```python
from build123d import *

# Parameters (mm, degrees)
EXTRUDE_1_DEPTH = 8


with BuildPart() as part:
    # 草图1 → 凸台-拉伸1 (new body)
    with BuildSketch(Plane.XY):
        with BuildLine():
            Line((9.884140627, 48.890967478), (9.862592606, 71.797167618))
            Line((9.862592606, 71.797167618), (9.862592606, 74.789638905))
            Line((9.862592606, 74.789638905), (1.859342158, 74.789638905))
            Line((1.859342158, 74.789638905), (1.859342158, 71.789638905))
            Line((1.859342158, 71.789638905), (1.880609299, 49.182021359))
            add(Edge.make_bspline(
                [(1.880609299, 49.182021359), (-2.147543525, 51.320103541), (-9.368620539, 54.40588996), (-18.684466246, 60.920686929), (-26.75654301, 68.367940859), (-36.33720868, 82.740540116), (-36.066485806, 97.042827626), (-36.847635358, 105.899002406)],
                knots=[0, 0, 0, 0, 0.18493282, 0.316628253, 0.458400557, 0.629057108, 1, 1, 1, 1], degree=3))
            Line((-36.847635358, 105.899002406), (47.833660698, 106.415821201))
            add(Edge.make_bspline(
                [(47.833660698, 106.415821201), (48.319473241, 99.869034947), (47.370463287, 91.039903293), (45.267329493, 80.35246618), (41.497074055, 73.927784135), (37.087778724, 67.31022324), (26.486440292, 57.93257211), (16.797369064, 52.799383097), (9.884140627, 48.890967478)],
                knots=[0, 0, 0, 0, 0.262570007, 0.359675169, 0.434109376, 0.560787033, 0.678988213, 1, 1, 1, 1], degree=3))
        make_face()
    extrude(amount=EXTRUDE_1_DEPTH)


solid = part.part
```
Verification items for the finished model (mm, model axes). Give positions to 0.01 mm unless a question says otherwise; leave off trailing zeros. Answer in a Markdown table with one row per item. Add a question column.
Item 1: Mould release check, pull along X, two halves, no side actions. Record for faces 1 (the flat face through (6, 74.79, 4)), 2 (the flat face through (6, 84, 8)): released by +X, released by -X, zero draft, split by the parting line, or undercut.
Item 2: Scan lines: probe 1 along X at (y, z) = (57, 2); probe 2 along X at (y, z) = (59, 3.75); probe 3 along X at (y, z) = (90, 6.5). Record each from-to range of solid material in increasing order. Write a range as from..to.
Item 3: Gauge pin test, flat ends, axial feed: pin 1 (0.9 mm diameter, centred on y = 73, z = 4, fed in from -X) (3 decimals); pin 2 (1.5 mm diameter, centred on y = 73.5, z = 5, fed in from +X); pin 3 (3 mm diameter, centred on y = 81, z = 2.5, fed in from -X). Record the tip position at first contact, or that the pin passes through.
Filled sheet:
| question | item | result |
|---|---|---|
| 1 | face 1 | undercut |
| 1 | face 2 | zero draft |
| 2 | probe 1 | x = -12.91..1.87, 9.88..23.83 |
| 2 | probe 2 | x = -15.81..1.87, 9.87..26.84 |
| 2 | probe 3 | x = -35.56..47 |
| 3 | pin 1 | stops at x = -29.935 |
| 3 | pin 2 | stops at x = 41.61 |
| 3 | pin 3 | stops at x = -34.04 |
